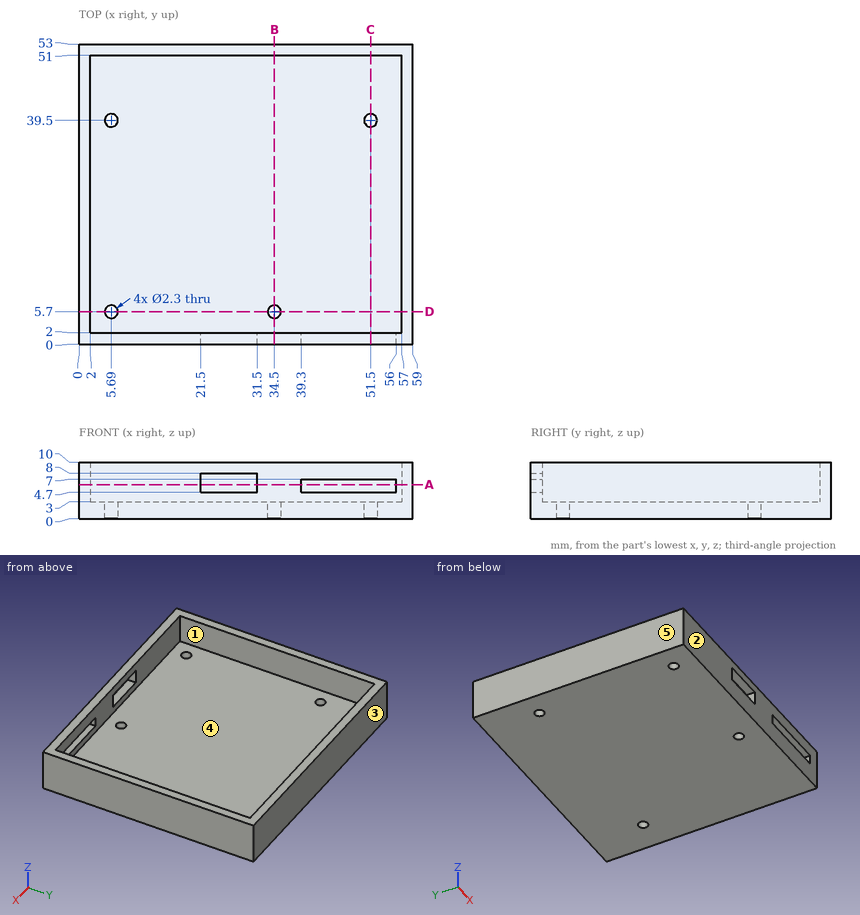
Verification items for this drawing (mm, ordinates from the low corner). A direction names the side the tool comes from. Round coordinates to 2 decimals unless told otherwise and drop trailing zeros. Order: outer loops, then holes, each group sorted by start corner. A loop starts at its lowest first (then second) coordinate and runs counter-clockwise, first axis right, second up.
1) Tool access check on the marked faces 1 and 2. Record the directions out of +Z, -Z, +X, -X, +Y, -Y that give a thin tool (end or side, any length) a straight path to the whole face; none if there is none.
Geometry says:
face 1: +Z
face 2: +Z, -Z, +X, -X, -Y
2) Cross-section at C-C, the plane x = 51.5. Record the cut outline in (y, z), plus the area to 4 significant figures.
Geometry says:
outline: (0, 0) - (38.35, 0) - (38.35, 3) - (2, 3) - (2, 4.7) - (0, 4.7) - close; (0, 7) - (2, 7) - (2, 10) - (0, 10) - close; (40.65, 0) - (53, 0) - (53, 10) - (51, 10) - (51, 3) - (40.65, 3) - close
area: 175.5 mm2
3) Material ranges on line 1 (Y direction, x = 5.69, z = 1.55); line 2 (Y direction, x = 5, z = 7); line 3 (X direction, y = 38, z = 4), recorded low to high.
Geometry says:
line 1: y = 0 to 4.55, 6.85 to 38.35, 40.65 to 53
line 2: y = 0 to 2, 51 to 53
line 3: x = 0 to 2, 57 to 59
4) Cross-section at D-D, the plane y = 5.7. Record the cut outline in (x, z).
Geometry says:
outline: (0, 0) - (4.54, 0) - (4.54, 3) - (2, 3) - (2, 10) - (0, 10) - close; (6.84, 0) - (33.35, 0) - (33.35, 3) - (6.84, 3) - close; (35.65, 0) - (59, 0) - (59, 10) - (57, 10) - (57, 3) - (35.65, 3) - close
5) Cross-section at B-B, the plane x = 34.5. Record the cut outline in (y, z).
Geometry says:
outline: (0, 0) - (4.55, 0) - (4.55, 3) - (2, 3) - (2, 10) - (0, 10) - close; (6.85, 0) - (53, 0) - (53, 10) - (51, 10) - (51, 3) - (6.85, 3) - close
6) Cross-section at A-A, the plane z = 6. Record the cut outline in (x, y).
Geometry says:
outline: (0, 0) - (21.5, 0) - (21.5, 2) - (2, 2) - (2, 51) - (57, 51) - (57, 2) - (56, 2) - (56, 0) - (59, 0) - (59, 53) - (0, 53) - close; (31.5, 0) - (39.3, 0) - (39.3, 2) - (31.5, 2) - close
7) Depth check by flat-ended pin: pin 1 (1.4 mm diameter, centred on x = 5.69, y = 5.7, fed in from -Z); pin 2 (3 mm diameter, centred on x = 5.69, y = 39.5, fed in from +Z). Enter the tip coordinate at first touch or a pass-through.
Geometry says:
pin 1: passes through
pin 2: stops at z = 3
8) Draft check along Y on the marked faces 3, 4 and 5. Enter one of: +Y half, -Y half, draft (parallel to the pull), parting line (faces both ways), or undercut.
Geometry says:
face 3: +Y half
face 4: undercut
face 5: draft
